The listing builds one solid part. Answer for the finished solid, in the listing's coordinates (mm). Coordinates: 2 decimals unless noted, no trailing zeros. Order: outer loops, then holes, each group sorted by start corner. A loop starts at its lowest first (then second) coordinate and runs counter-clockwise, first axis right, second up.
from build123d import *

# Parameters (mm, degrees)
F0_R     = 76.2
F1_DEPTH = 25.4
F3_D     = 139.7
F4_R     = 69.85
F5_DEPTH = 25.4
F7_D     = 127


with BuildPart() as f1:
    # F0 (on Front) → F1 (new body)
    with BuildSketch(Plane.XZ):
        with Locations((-6.108229, 2.87896)):
            Circle(F0_R)
    extrude(amount=F1_DEPTH)

    # F3 (through all)
    with Locations(Plane.XZ):
        with Locations((-6.108229, 2.87896)):
            Hole(F3_D / 2)

    # F4 (on Front) → F5 (join)
    with BuildSketch(Plane.XZ):
        with Locations((-74.529298, 67.110427)):
            Circle(F4_R)
    extrude(amount=F5_DEPTH)

    # F7 (through all)
    with Locations(Plane.XZ.offset(25.4)):
        with Locations((-74.529298, 67.110427)):
            Hole(F7_D / 2)


solid = f1.part
(1) Find section C-C on y = -14.5. Determine the outline of the cut face in (x, z), then the cut area to 3 significant figures.
(2) Find section B-B on z = 31. Determine the outline of the cut face in (x, y).
(3) Given pin 1 Ø4 at (y, z) = (-6, 75.5) entering from -X; pin 2 Ø1 at (y, z) = (-15.5, 51) entering from +X; pin 3 Ø12 at (x, y) = (-16.5, -17) entering from +Z, each flat-ended and moving along its own axis, determine where each tip first touches the part or whether it passes through.
(4) Find section A-A on x = -88. Determine the outline of the cut face in (y, z), then the cut area to 3 significant figures.
(5) Find section D-D on x = -19. Determine the outline of the cut face in (y, z), then the cut area to 3 significant figures.
(6) The mould has two halves that part along X. Classify faces 1 (the cylindrical face through (-24.165, -12.522, 18.711)), 2 (the cylindrical face through (-123.95, -12.52, 116.47)), 3 (the flat face through (-30, -25.4, 17)): pulls with the +X half, pulls with the -X half, needs draft (parallel to the pull), parting line crosses it, or undercut.
(7) Find the intervals of material crossed by probe 1 along Z at (x, y) = (-25, -12.25); probe 2 along Z at (x, y) = (-46.5, -21.5); probe 3 along X at (y, z) = (-17.5, 41), in increasing order.
Resolved:
1. outline: (-82.13, -2.32) arc R76.2 ccw (long way) to (-5.71, 79.08) arc R69.85 ccw (long way) to start; hole circle Ø127 at (-74.53, 67.11); hole (-75.73, -2.73) arc R69.85 ccw (long way) to (-4.9, 72.72) arc R69.85 cw to start
1. area: 4,810 mm2
2. outline: (-134.32, -25.4) - (-126.76, -25.4) - (-126.76, 0) - (-134.32, 0) - close; (-22.3, -25.4) - (-14.74, -25.4) - (-14.74, 0) - (-22.3, 0) - close; (57.83, -25.4) - (64.71, -25.4) - (64.71, 0) - (57.83, 0) - close
3. pin 1: stops at x = -144.09
3. pin 2: stops at x = 53.38
3. pin 3: stops at z = 113.71
4. outline: (-25.4, -1.43) - (0, -1.43) - (0, 5.06) - (-25.4, 5.06) - close; (-25.4, 129.17) - (0, 129.17) - (0, 135.65) - (-25.4, 135.65) - close
4. area: 329 mm2
5. outline: (-25.4, -72.22) - (0, -72.22) - (0, -65.77) - (-25.4, -65.77) - close; (-25.4, 24.74) - (0, 24.74) - (0, 36.31) - (-25.4, 36.31) - close; (-25.4, 97.91) - (0, 97.91) - (0, 109.48) - (-25.4, 109.48) - close
5. area: 752 mm2
6. face 1: undercut
6. face 2: parting line crosses it
6. face 3: needs draft
7. probe 1: z = -70.94 to -64.37, 17.86 to 27.37, 106.85 to 116.36
7. probe 2: z = -61.73 to -54.11, 3.13 to 10.13, 124.09 to 131.09
7. probe 3: x = -139.32 to -132.41, -16.65 to -9.74, 52.42 to 59.87
